Check sheet for the modelled part. Datum: model origin and axes. Units: mm. A direction names the side the tool comes from. Coordinates: 2 decimals unless noted, no trailing zeros. Write each loop counter-clockwise with the first axis right and the second up, starting at its lowest first coordinate (ties: lowest second). Pieces come first, ordered by that corner, then holes. Notation, with made-up numbers: (48, 37) - (64, 37) arc R13 cw to (64, 62) - close; hole circle Ø11 at (85.5, 50). An arc over 180 degrees is marked (long way). Write each question's results on one line, items separated by ' | '.
Autodesk Inventor part; units mm, degrees
ref_plane "YZ Plane" through (0, 0, 0) normal (1, 0, 0) x (0, 1, 0)
ref_plane "XZ Plane" through (0, 0, 0) normal (0, 1, 0) x (-1, 0, 0)
ref_plane "XY Plane" through (0, 0, 0) normal (0, 0, 1) x (1, 0, 0)
sketch "Sketch1" plane through (0, 0, 0) normal (0, 1, 0) x (-1, 0, 0)
  line L0 (17.0295, 14.999) -> (-8.3705, 14.999)
  line L1 (-8.3705, 14.999) -> (-8.3705, -10.401)
  line L2 (-8.3705, -10.401) -> (17.0295, -10.401)
  line L3 (17.0295, -10.401) -> (17.0295, 14.999)
  line L4 (15.442, -8.8135) -> (-6.783, -8.8135)
  line L5 (-6.783, -8.8135) -> (-6.783, 13.4115)
  line L6 (-6.783, 13.4115) -> (15.442, 13.4115)
  line L7 (15.442, 13.4115) -> (15.442, -8.8135)
  point P0 (0, 0)
  dimension "d0" = 25.4
  dimension "d1" = 25.4
  dimension "d4" = 1.5875
  dimension "d5" = 1.5875
  dimension "d6" = 1.5875
  dimension "d7" = 1.5875
extrude "Extrusion2" add sketch "Sketch1" along normal blind 990.6
sketch "Sketch5" plane through (8.3705, 0, 14.999) normal (1, 0, 0) x (0, 0, -1)
  line L0 (0, 0) -> (0, 990.6)
  line L1 (0, 0) -> (25.4, 0)
  point P0 (14.999, 0)
  point P1 (12.7, 38.1)
  dimension "d37" = 12.7
  dimension "d38" = 38.1
hole "Hole4" at (8.3705, 38.1, 2.299) direction (-1, 0, 0) diameter 9.5758 depth 25.4 tip angle 118
sketch "Sketch6" plane through (8.3705, 0, 14.999) normal (1, 0, 0) x (0, 0, -1)
  line L0 (25.4, 0) -> (25.4, 990.6)
  line L1 (0, 990.6) -> (25.4, 990.6)
  point P0 (14.999, 0)
  point P1 (12.7, 952.5)
  dimension "d46" = 12.7
  dimension "d47" = 38.1
hole "Hole5" at (8.3705, 952.5, 2.299) direction (-1, 0, 0) diameter 9.5758 depth 25.4 tip angle 118
sketch "Sketch7" plane through (8.3705, 0, 14.999) normal (1, 0, 0) x (0, 0, -1)
  line L0 (0, 0) -> (0, 990.6)
  line L1 (0, 0) -> (25.4, 0)
  point P0 (14.999, 0)
  point P1 (12.7, 101.6)
  point P2 (12.7, 127)
  point P3 (12.7, 152.4)
  dimension "d55" = 12.7
  dimension "d56" = 0
  dimension "d57" = 0
  dimension "d58" = 101.6
  dimension "d59" = 25.4
  dimension "d60" = 25.4
hole "Hole6" at (8.3705, 101.6, 2.299) at (8.3705, 127, 2.299) at (8.3705, 152.4, 2.299) direction (-1, 0, 0) diameter 4.826 depth 25.4 tip angle 118
sketch "Sketch8" plane through (8.3705, 0, 14.999) normal (1, 0, 0) x (0, 0, -1)
  line L0 (0, 990.6) -> (25.4, 990.6)
  line L1 (0, 0) -> (0, 990.6)
  point P0 (14.999, 0)
  point P1 (12.7, 914.4)
  point P2 (12.7, 889)
  point P3 (12.7, 863.6)
  dimension "d68" = 76.2
  dimension "d69" = 25.4
  dimension "d70" = 25.4
  dimension "d71" = 12.7
  dimension "d72" = 0
  dimension "d73" = 0
hole "Hole7" at (8.3705, 914.4, 2.299) at (8.3705, 889, 2.299) at (8.3705, 863.6, 2.299) direction (-1, 0, 0) diameter 4.826 depth 25.4 tip angle 118
sketch "Sketch9" plane through (-17.0295, 0, 14.999) normal (0, 0, 1) x (1, 0, 0)
  line L0 (25.4, 0) -> (25.4, 990.6)
  line L1 (0, 0) -> (0, 990.6)
  line L2 (0, 990.6) -> (25.4, 990.6)
  point P0 (17.0295, 0)
  point P1 (6.35, 971.55)
  point P2 (19.05, 984.25)
  point P3 (6.35, 946.15)
  point P4 (19.05, 958.85)
  dimension "d81" = 6.35
  dimension "d82" = 6.35
  dimension "d83" = 6.35
  dimension "d84" = 6.35
  dimension "d85" = 25.4
  dimension "d86" = 25.4
  dimension "d87" = 6.35
  dimension "d88" = 19.05
hole "Hole8" at (-10.6795, 971.55, 14.999) at (2.0205, 984.25, 14.999) at (-10.6795, 946.15, 14.999) at (2.0205, 958.85, 14.999) direction (0, 0, -1) diameter 4.7625 depth 25.4 tip angle 118
sketch "Sketch10" plane through (-17.0295, 0, 14.999) normal (0, 0, 1) x (1, 0, 0)
  line L0 (25.4, 0) -> (25.4, 990.6)
  line L1 (0, 0) -> (25.4, 0)
  line L2 (0, 0) -> (0, 990.6)
  point P0 (17.0295, 0)
  point P1 (19.05, 44.45)
  point P2 (19.05, 69.85)
  point P3 (6.35, 31.75)
  point P4 (6.35, 57.15)
  dimension "d96" = 6.35
  dimension "d97" = 6.35
  dimension "d98" = 25.4
  dimension "d99" = 44.45
  dimension "d100" = 6.35
  dimension "d101" = 31.75
  dimension "d102" = 6.35
  dimension "d103" = 25.4
hole "Hole9" at (2.0205, 44.45, 14.999) at (2.0205, 69.85, 14.999) at (-10.6795, 31.75, 14.999) at (-10.6795, 57.15, 14.999) direction (0, 0, -1) diameter 4.7625 depth 25.4 tip angle 118
equation "\"d0\" = ElvBeamWidth"
equation "\"d1\" = ElvBeamWidth"
equation "\"d4\" = ElvWallWidth"
equation "\"d5\" = ElvWallWidth"
equation "\"d6\" = ElvWallWidth"
equation "\"d7\" = ElvWallWidth"
equation "\"d8\" = ElvFixedBeamLength"
equation "\"ElvMiddleBeamLength\" = 990.6"
equation "\"ElvWallWidth\" = 1.5875"
equation "\"ElvFrontBeamLength\" = 990.6"
equation "\"ElvEndEffectLength\" = 431.8"
equation "\"ElvCrossBeamLength\" = 304.8"
equation "\"ElvBeamWidth\" = 25.4"
equation "\"ElvFrontBeamLength_1\" = 1066.8"
equation "\"ElvFixedBeamLength\" = 990.6"
equation "\"ElvDelDepth\" = 6.35"
equation "\"ElvDelWidth\" = 18.542"
equation "\"ElvDelFrontTabLength\" = 6.35"
equation "\"ElvDelHeight\" = 101.6"
equation "\"ElvTopBeamLength\" = 457.2"
equation "\"ElvHoleFromBottom\" = 38.1"
equation "\"ElvHoleFromFixed\" = 50.8"
equation "\"ElvHoleFromMid\" = 38.1"
equation "\"ElvHoleFromFront\" = 25.4"
equation "\"ElvRivetPlateLength\" = 76.2"
equation "\"ElvDelMiddleTabLength\" = 6.35"
properties part number "ElvMiddleBeam"
1. Sectioned sample at A-A (y = 639.5). Record the cut outline in (x, z).
Values follow:
outline: (-17.03, -10.4) - (8.37, -10.4) - (8.37, 15) - (-17.03, 15) - close; hole (-15.44, -8.81) - (6.78, -8.81) - (6.78, 13.41) - (-15.44, 13.41) - close
2. Access from +Z, -Z, +X, -X, +Y, -Y to the whole of each face (thin tool, end or side, straight path). Record for faces 5 (the flat face through (-15.442, 488, 2)), 6 (the flat face through (8.37, 488, 2)).
Values follow:
face 5: +Y, -Y | face 6: +Z, -Z, +X, +Y, -Y
3. Material ranges on L1, parallel to Z at x = 3.75, y = 183; L2, parallel to X at y = 625, z = 6.5; L3, parallel to X at y = 946.15, z = -9.9, recorded low to high. Write a range as [from, to].
Values follow:
L1: z = [-10.4, -8.81], [13.41, 15] | L2: x = [-17.03, -15.44], [6.78, 8.37] | L3: x = [-17.03, -13.06], [-8.3, 8.37]
4. Draft check along Z on faces 1 (the flat face through (-4, 488, -10.401)), 2 (the flat face through (-17.03, 488, 2)), 3 (the flat face through (6.783, 488, 2)), 4 (the flat face through (-5, 488, 14.999)). Enter one of: pulls with the +Z half, pulls with the -Z half, needs draft (parallel to the pull), parting line crosses it, or undercut.
Values follow:
face 1: pulls with the -Z half | face 2: needs draft | face 3: undercut | face 4: pulls with the +Z half
5. Go/stop test with a flat-tipped pin: pin 1 (7.5 mm diameter, centred on y = 914.4, z = 2.299, fed in from +X). Record where the tip stops, or that it passes through.
Values follow:
pin 1: stops at x = 8.37
